Read the model definition and answer for the solid it produces. Units are mm, in the model's axes. Face numbers are marked on the shaded views. A direction names the side the tool comes from. Coordinates: 2 decimals unless noted, no trailing zeros. Write each loop counter-clockwise with the first axis right and the second up, starting at its lowest first coordinate (ties: lowest second). Pieces come first, ordered by that corner, then holes.
Item 1: Each of these flat-tipped pins is pushed along its axis until it touches: P1, Ø1.5, axis at x = 10.5, y = 0, coming from the +Z side; P2, Ø4, axis at x = 19, z = -3.5, coming from the -Y side; P3, Ø0.6, axis at y = -2, z = 1, coming from the -X side. Where does it stop, or does it pass through?
Item 2: Straight lines are drawn through the part: probe 1 along Y at (x, z) = (5.95, 0); probe 2 along X at (y, z) = (-3.5, -1.75); probe 3 along Z at (x, y) = (5.5, 4). For each, find the intervals that lie inside material, in ascending order.
Item 3: A tool of negligible diameter and unlimited length cuts with its end or side. For the marked faces 5 and 6, from which of +Z, -Z, +X, -X, +Y, -Y can it reach the whole face along a straight path? Write none if from no direction.
Item 4: Determine the mould class of the marked faces 1, 2, 3 and 4 for opening direction Y: released by +Y, released by -Y, zero draft, split by the parting line, or undercut.
Item 5: Section A-A (x = 2.5) is taken. Give the vertices of the cut face in (y, z), then the cut area to 3 significant figures.
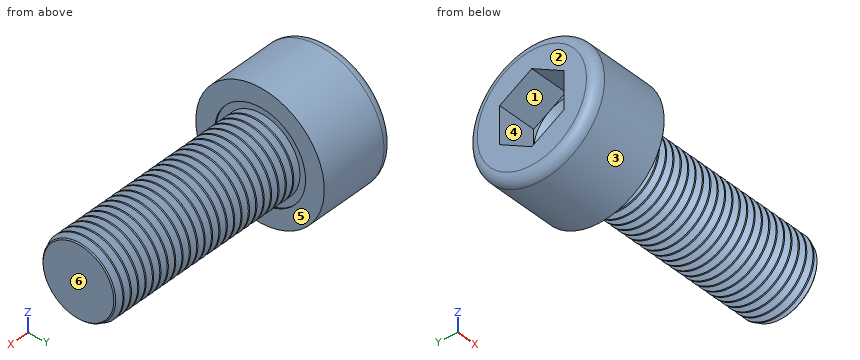
from build123d import *

# Parameters (mm, degrees)
SKETCH1_R           = 5
BASEHEAD_DEPTH      = 6
SKETCH2_R           = 3
BASEBODY_DEPTH      = 16
HEXAGONSOCKET_DEPTH = 3
TOPFILLET_R         = 0.75
CHAMFER1_SIZE       = 0.25
LPATTERN10_COUNT    = 25
LPATTERN10_PITCH    = 0.6498


with BuildPart() as part:
    # Sketch1 → BaseHead (new body)
    with BuildSketch(Plane(origin=(0, 0, 0), x_dir=(0, 0, -1), z_dir=(1, 0, 0))):
        Circle(SKETCH1_R)
    extrude(amount=BASEHEAD_DEPTH)

    # Sketch2 → BaseBody (add)
    with BuildSketch(Plane(origin=(6, 0, 0), x_dir=(0, 0, -1), z_dir=(1, 0, 0))):
        Circle(SKETCH2_R)
    extrude(amount=BASEBODY_DEPTH)

    # Sketch3 → HexagonSocket (cut)
    with BuildSketch(Plane(origin=(0, 0, 0), x_dir=(0, 0, -1), z_dir=(1, 0, 0))):
        Polygon((2.886751346, 0), (1.443375673, 2.5), (-1.443375673, 2.5), (-2.886751346, 0), (-1.443375673, -2.5), (1.443375673, -2.5), align=None)
    extrude(amount=HEXAGONSOCKET_DEPTH, mode=Mode.SUBTRACT)

    # Sketch4 → Cut-Revolve1 (revolve, cut)
    with BuildSketch(Plane(origin=(-4.19613823, 0.75, 0), x_dir=(-1, 0, 0), z_dir=(0, 0, 1))):
        Polygon((-7.19613823, 3.25), (-8.639513903, 0.75), (-7.19613823, 0.75), align=None)
    revolve(axis=Axis((0.838992387, 0, 0), (-1, 0, 0)), mode=Mode.SUBTRACT)

    # TopFillet
    topfillet_edges = [part.edges().sort_by_distance(p)[0] for p in [
        (0, 0, 5),
    ]]
    fillet(topfillet_edges, radius=TOPFILLET_R)

    # Chamfer1
    chamfer1_edges = [part.edges().sort_by_distance(p)[0] for p in [
        (22, 0, 3),
    ]]
    chamfer(chamfer1_edges, length=CHAMFER1_SIZE)

    # Sketch5 → Cut-Revolve10 (revolve, cut)
    with BuildSketch(Plane.XY):
        Polygon((21.75, 2.531047244), (22.02075, 3), (22.02075, 3.5415), (21.47925, 3.5415), (21.47925, 3), align=None)
    cut_revolve10 = revolve(axis=Axis((0, 0, 0), (1, 0, 0)), mode=Mode.SUBTRACT)

    # LPattern10: Cut-Revolve10 ×25
    with Locations(*[(-i * LPATTERN10_PITCH, 0, 0) for i in range(1, LPATTERN10_COUNT)]):
        add(cut_revolve10, mode=Mode.SUBTRACT)


solid = part.part
Established:
1. P1: stops at z = 3
1. P2: stops at y = -2.6
1. P3: stops at x = 3
2. probe 1: y = -5 to -3.54, -2.89 to 2.89, 3.54 to 5
2. probe 2: x = 0 to 6
2. probe 3: z = -3 to 3
3. face 5: +X
3. face 6: +Z, -Z, +X, +Y, -Y
4. face 1: undercut
4. face 2: zero draft
4. face 3: split by the parting line
4. face 4: undercut
5. outline: circle Ø10 at (0, 0); hole (-2.5, -1.44) - (0, -2.89) - (2.5, -1.44) - (2.5, 1.44) - (0, 2.89) - (-2.5, 1.44) - close
5. area: 56.9 mm2
